Design review of the part built by this model. Coordinates are the model's own, in mm. Face numbers are marked on the shaded views. A direction names the side the tool comes from. Give positions to 0.01 mm unless a question says otherwise; leave off trailing zeros. Order: outer loops, then holes, each group sorted by start corner. A loop starts at its lowest first (then second) coordinate and runs counter-clockwise, first axis right, second up.
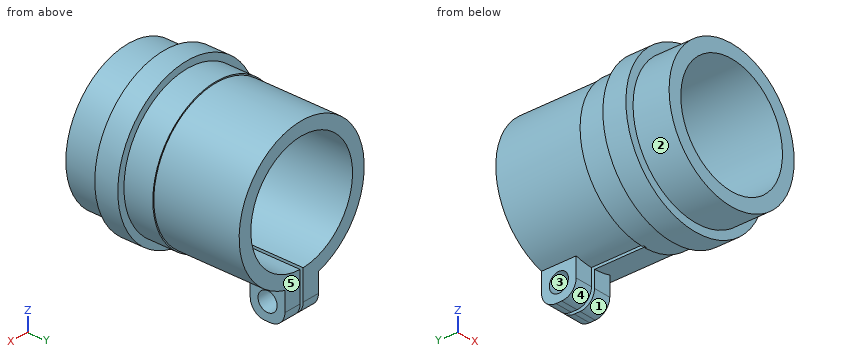
```python
from build123d import *

# Parameters (mm, degrees)
SKETCH1_R           = 15.875
SKETCH1_R_2         = 12.7
BOSS_EXTRUDE1_DEPTH = 38.1
SKETCH2_R           = 17.399
SKETCH2_R_2         = 15.875
BOSS_EXTRUDE2_DEPTH = 5.0673
SKETCH3_R           = 15.875
SKETCH3_R_2         = 15.621
CUT_EXTRUDE1_DEPTH  = 7.9248
CUT_EXTRUDE2_START  = -19.3421
SKETCH3_2_R         = 15.875
SKETCH3_2_R_2       = 15.621
CUT_EXTRUDE2_DEPTH  = 18.7579
SKETCH4_W           = 0.762
SKETCH4_H           = 4.704716286
CUT_EXTRUDE3_DEPTH  = 19.05
SKETCH5_W           = 9.757521138
SKETCH5_H           = 7.62
SKETCH5_R           = 2.1
BOSS_EXTRUDE3_DEPTH = 3.81
FILLET1_R           = 3.175


with BuildPart() as part:
    # Sketch1 → Boss-Extrude1 (new body)
    with BuildSketch(Plane(origin=(0, 0, 0), x_dir=(1, 0, 0), z_dir=(0, 1, 0))):
        with Locations(Location((0, 0, 0), (0, 0, 90))):
            Circle(SKETCH1_R)
        with Locations(Location((0, 0, 0), (0, 0, 90))):
            Circle(SKETCH1_R_2, mode=Mode.SUBTRACT)
    extrude(amount=BOSS_EXTRUDE1_DEPTH)

    # Sketch2 → Boss-Extrude2 (add)
    with BuildSketch(Plane(origin=(0, 7.9248, 0), x_dir=(-1, 0, 0), z_dir=(0, -1, 0))):
        with Locations(Location((0, 0, 0), (0, 0, 90))):
            Circle(SKETCH2_R)
        with Locations(Location((0, 0, 0), (0, 0, 90))):
            Circle(SKETCH2_R_2, mode=Mode.SUBTRACT)
    extrude(amount=-BOSS_EXTRUDE2_DEPTH)

    # Sketch3 → Cut-Extrude1 (cut)
    with BuildSketch(Plane.XZ):
        with Locations(Location((0, 0, 0), (0, 0, 270))):
            Circle(SKETCH3_R)
        with Locations(Location((0, 0, 0), (0, 0, 270))):
            Circle(SKETCH3_R_2, mode=Mode.SUBTRACT)
    extrude(amount=-CUT_EXTRUDE1_DEPTH, mode=Mode.SUBTRACT)

    # Sketch3<2> → Cut-Extrude2 (cut)
    with BuildSketch(Plane.XZ.offset(CUT_EXTRUDE2_START)):
        with Locations(Location((0, 0, 0), (0, 0, 270))):
            Circle(SKETCH3_2_R)
        with Locations(Location((0, 0, 0), (0, 0, 270))):
            Circle(SKETCH3_2_R_2, mode=Mode.SUBTRACT)
    extrude(amount=-CUT_EXTRUDE2_DEPTH, mode=Mode.SUBTRACT)

    # Sketch4 → Cut-Extrude3 (cut)
    with BuildSketch(Plane(origin=(0, 38.1, 0), x_dir=(1, 0, 0), z_dir=(0, 1, 0))):
        with Locations((0, 15.046641857)):
            Rectangle(SKETCH4_W, SKETCH4_H)
    extrude(amount=-CUT_EXTRUDE3_DEPTH, mode=Mode.SUBTRACT)

    # Sketch5 → Boss-Extrude3 (add)
    with BuildSketch(Plane.ZY.offset(-0.381)):
        with Locations((-17.573044283, 34.29)):
            Rectangle(SKETCH5_W, SKETCH5_H)
        with Locations((-18.641804852, 34.29)):
            Circle(SKETCH5_R, mode=Mode.SUBTRACT)
    boss_extrude3 = extrude(amount=-BOSS_EXTRUDE3_DEPTH)

    # Mirror1: Boss-Extrude3 across plane
    add(boss_extrude3.mirror(Plane(origin=(0, 0, 0), x_dir=(0, 0, 1), z_dir=(1, 0, 0))))

    # Fillet1
    fillet1_edges = [part.edges().sort_by_distance(p)[0] for p in [
        (-2.286, 30.48, -22.451804852),
        (2.286, 30.48, -22.451804852),
        (2.286, 38.1, -22.451804852),
        (-2.286, 38.1, -22.451804852),
    ]]
    fillet(fillet1_edges, radius=FILLET1_R)


solid = part.part
```
1. Take a section at C-C (x = -8). State the section outline as (y, z) points, then the cut area to 3 significant figures.
Recorded:
outline: (0, -13.42) - (7.92, -13.42) - (7.92, -15.45) - (12.99, -15.45) - (12.99, -13.71) - (19.34, -13.71) - (19.34, -13.42) - (38.1, -13.42) - (38.1, -9.86) - (0, -9.86) - close; (0, 9.86) - (38.1, 9.86) - (38.1, 13.42) - (19.34, 13.42) - (19.34, 13.71) - (12.99, 13.71) - (12.99, 15.45) - (7.92, 15.45) - (7.92, 13.42) - (0, 13.42) - close
area: 295 mm2
2. Take a section at A-A (z = 0). State the section outline as (x, y) points (3 decimals), then the cut area to 3 significant figures.
Recorded:
outline: (-17.399, 7.925) - (-15.621, 7.925) - (-15.621, 0) - (-12.7, 0) - (-12.7, 38.1) - (-15.621, 38.1) - (-15.621, 19.342) - (-15.875, 19.342) - (-15.875, 12.992) - (-17.399, 12.992) - close; (12.7, 0) - (15.621, 0) - (15.621, 7.925) - (17.399, 7.925) - (17.399, 12.992) - (15.875, 12.992) - (15.875, 19.342) - (15.621, 19.342) - (15.621, 38.1) - (12.7, 38.1) - close
area: 244 mm2
3. Draft analysis for pull direction Z (two halves, no side actions). For the marked faces 3, 4 and 5, state which applies: pulls with the +Z half, pulls with the -Z half, needs draft (parallel to the pull), parting line crosses it, or undercut.
Recorded:
face 3: undercut
face 4: pulls with the -Z half
face 5: needs draft
4. For pin 1 (17.5 mm diameter, centred on x = 8.5, z = 1.5, fed in from -Y); pin 2 (1.9 mm diameter, centred on x = 2, z = -17.5, fed in from -Y); pin 3 (4 mm diameter, centred on y = 31, z = 12.5, fed in from -X); pin 4 (5 mm diameter, centred on y = 33, z = -16, fed in from +X), all flat-tipped, find the tip position at first contact; note any pin that passes through.
Recorded:
pin 1: stops at y = 0
pin 2: stops at y = 7.92
pin 3: stops at x = -11.57
pin 4: stops at x = 7.86
5. Take a section at D-D (y = 8.5). State the section outline as (x, z) points.
Recorded:
outline: circle Ø34.8 at (0, 0); hole circle Ø25.4 at (0, 0)
6. For line 1 along X through (y, z) = (24, 0); line 2 along X through (y, z) = (6, -7); line 3 along Z through (x, y) = (-3, 3), list the stretches that pass through material, from the lowest coordinate up.
Recorded:
line 1: x = -15.62 to -12.7, 12.7 to 15.62
line 2: x = -13.96 to -10.6, 10.6 to 13.96
line 3: z = -15.33 to -12.34, 12.34 to 15.33
7. Machinability: for the marked faces 1 and 2, which of the approach directions +Z, -Z, +X, -X, +Y, -Y give a long, thin tool a straight path to every point of the face, cutting with its end or side? Answer none if there is none.
Recorded:
face 1: -Z, +X, -X, -Y
face 2: -Y
8. Take a section at B-B (y = 34.29). State the section outline as (x, z) points, then the cut area to 3 significant figures.
Recorded:
outline: (-4.19, -22.45) - (-0.38, -22.45) - (-0.38, -20.74) - (-4.19, -20.74) - close; (-4.19, -16.54) - (-0.38, -16.54) - (-0.38, -12.69) arc R12.7 cw (long way) to (0.38, -12.69) - (0.38, -16.54) - (4.19, -16.54) - (4.19, -15.05) arc R15.62 ccw (long way) to (-4.19, -15.05) - close; (0.38, -22.45) - (4.19, -22.45) - (4.19, -20.74) - (0.38, -20.74) - close
area: 279 mm2
